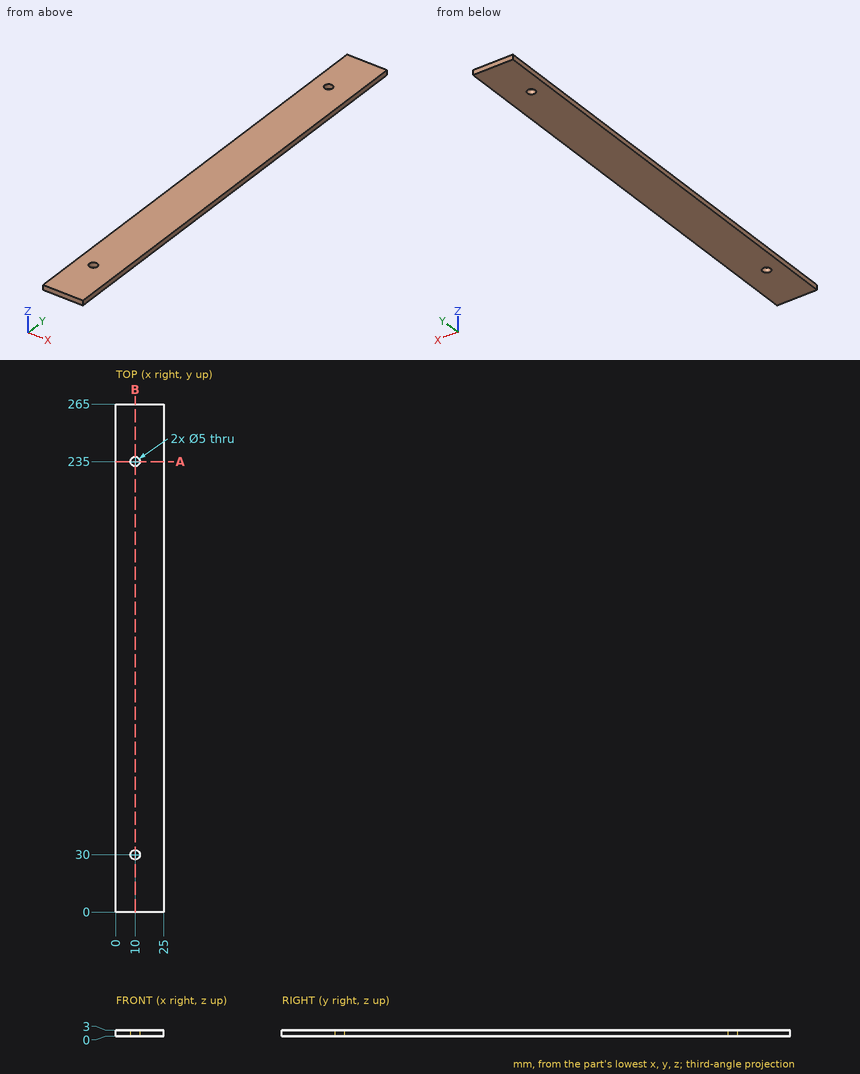
Input: dimensioned drawing with shaded views. Units: mm. Origin: part minimum x, y, z. Round coordinates to 2 decimals unless told otherwise and drop trailing zeros. Order: outer loops, then holes, each group sorted by start corner. A loop starts at its lowest first (then second) coordinate and runs counter-clockwise, first axis right, second up. Notation, with made-up numbers: (86, -30) - (90, -30) arc R18 ccw to (90, -26) - close; hole circle Ø7 at (40, 50). An arc over 180 degrees is marked (long way). Write item = value, one per line. Start each with the question number.
Q1. Cut plane A-A on y = 235. Return the cut outline in (x, z).
Q2. Cut plane B-B on x = 10. Return the cut outline in (y, z), and give its area (3 significant figures).
Q3. Ray query, line 1 (Y direction, x = 10, z = 1.95); line 2 (X direction, y = 30, z = 2.15); line 3 (Y direction, x = 11.75, z = 1.7). Return the intervals inside material, ascending. Write a range as from..to.
Outcome:
q1.outline = (0, 0) - (7.5, 0) - (7.5, 3) - (0, 3) - close; (12.5, 0) - (25, 0) - (25, 3) - (12.5, 3) - close
q2.outline = (0, 0) - (27.5, 0) - (27.5, 3) - (0, 3) - close; (32.5, 0) - (232.5, 0) - (232.5, 3) - (32.5, 3) - close; (237.5, 0) - (265, 0) - (265, 3) - (237.5, 3) - close
q2.area = 765 mm^2
q3.line_1 = 0..27.5, 32.5..232.5, 237.5..265
q3.line_2 = 0..7.5, 12.5..25
q3.line_3 = 0..28.21, 31.79..233.21, 236.79..265
